from build123d import *

# Parameters (mm, degrees)
F0_W     = 157.5113609433
F0_H     = 71.6332271695
F1_DEPTH = 40
F2_R     = 5
F3_R     = 26.0186453027
F4_DEPTH = 20
F5_W     = 51.7887976021
F5_H     = 11.637929827
F6_DEPTH = 35
F7_R     = 5


# Not quite as in the source:
# - the program builds the solid bodies; features that only make, move or delete a surface that nothing else refers to are left out


with BuildPart() as f1:
    # F0 (on Front) → F1 (new body)
    with BuildSketch(Plane.XZ):
        with Locations((3.7253e-06, 35.8166135848)):
            Rectangle(F0_W, F0_H)
    extrude(amount=F1_DEPTH)

    # F2
    f2_edges = [f1.edges().sort_by_distance(p)[0] for p in [
        (4e-06, -40, 71.633227),
        (4e-06, 0, 71.633227),
        (78.755684, -40, 35.816614),
        (78.755684, 0, 35.816614),
        (78.755684, -20, 71.633227),
        (-78.755677, -20, 71.633227),
        (-78.755677, 0, 35.816614),
        (-78.755677, -40, 35.816614),
    ]]
    fillet(f2_edges, radius=F2_R)

    # F3 (on face) → F4 (cut)
    with BuildSketch(Plane.XZ.offset(40)):
        with Locations((-36.0129252076, 33.036891371)):
            Circle(F3_R)
    extrude(amount=-F4_DEPTH, mode=Mode.SUBTRACT)

    # F5 (on face) → F6 (cut)
    with BuildSketch(Plane.XY.offset(71.6332271695)):
        with Locations((-6.1099091545, -19.590517506)):
            Rectangle(F5_W, F5_H)
    extrude(amount=-F6_DEPTH, mode=Mode.SUBTRACT)

    # F7
    f7_edges = [f1.edges().sort_by_distance(p)[0] for p in [
        (4e-06, -40, 0),
    ]]
    fillet(f7_edges, radius=F7_R)


solid = f1.part
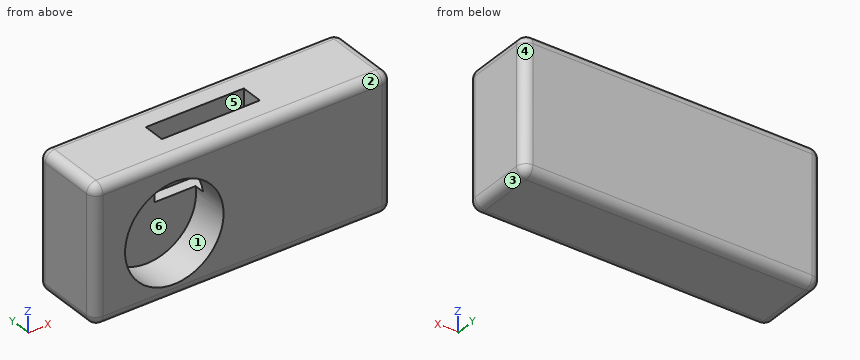
The listing builds one solid part. Answer for the finished solid, in the listing's coordinates (mm). Face numbers are marked on the shaded views. A direction names the side the tool comes from. Give positions to 0.01 mm unless a question says otherwise; leave off trailing zeros. Order: outer loops, then holes, each group sorted by start corner. A loop starts at its lowest first (then second) coordinate and runs counter-clockwise, first axis right, second up. Notation, with made-up numbers: (74.5, 61.25) - (89.5, 61.25) arc R17 cw to (89.5, 88.25) - close; hole circle Ø11 at (-19, 79). An arc over 180 degrees is marked (long way). One line per item, written item: value. Start each with the question number.
1) A cutting plane is placed at C-C on x = -1. Give the vertices of the cut face in (y, z), then the cut area to 3 significant figures.
2) A cutting plane is placed at B-B on y = -33.5. Give the vertices of the cut face in (x, z).
3) The mould has two halves that part along Y. Classify the marked faces 3, 4, 5 and 6: released by +Y, released by -Y, zero draft, split by the parting line, or undercut.
4) Find the intervals of material crossed by L1, parallel to X at y = -19, z = 40; L2, parallel to Y at x = -38.5, z = 13; L3, parallel to X at y = -4.5, z = 38, in increasing order.
5) A tool of negligible diameter and unlimited length cuts with its end or side. For the marked faces 1 and 2, from which of +Z, -Z, +X, -X, +Y, -Y can it reach the whole face along a straight path? Write none if from no direction.
6) Given pin 1 Ø3.5 at (x, y) = (-4.5, -18) entering from +Z; pin 2 Ø5 at (x, z) = (-26.5, 44.5) entering from -Y; pin 3 Ø15.5 at (x, z) = (-25, 31.5) entering from -Y, each flat-ended and moving along its own axis, determine where each tip first touches the part or whether it passes through.
7) A cutting plane is placed at A-A on x = -19.5. Give the vertices of the cut face in (y, z).
8) A cutting plane is placed at D-D on y = -16.5. Give the vertices of the cut face in (x, z).
Answer sheet:
1. outline: (-40, 5) arc R5 ccw to (-35, 0) - (-5, 0) arc R5 ccw to (0, 5) - (0, 66.63) arc R5 ccw to (-5, 71.63) - (-13.77, 71.63) - (-13.77, 36.63) - (-25.41, 36.63) - (-25.41, 71.63) - (-35, 71.63) arc R5 ccw to (-40, 66.63) - close
1. area: 2,440 mm2
2. outline: (-78.76, 5) arc R5 ccw to (-73.76, 0) - (73.76, 0) arc R5 ccw to (78.76, 5) - (78.76, 66.63) arc R5 ccw to (73.76, 71.63) - (-73.76, 71.63) arc R5 ccw to (-78.76, 66.63) - close; hole circle Ø52.04 at (-36.01, 33.04)
3. face 3: zero draft
3. face 4: released by +Y
3. face 5: undercut
3. face 6: released by -Y
4. L1: x = -78.76 to -32, 19.78 to 78.76
4. L2: y = -20 to 0
4. L3: x = -78.73 to 78.73
5. face 1: -Y
5. face 2: +Z, +X, -X, -Y
6. pin 1: stops at z = 36.63
6. pin 2: stops at y = -13.77
6. pin 3: stops at y = -20
7. outline: (-40, 5) arc R5 ccw to (-35, 0) - (-5, 0) arc R5 ccw to (0, 5) - (0, 66.63) arc R5 ccw to (-5, 71.63) - (-13.77, 71.63) - (-13.77, 36.63) - (-20, 36.63) - (-20, 12.93) - (-40, 12.93) - close; (-40, 53.14) - (-25.41, 53.14) - (-25.41, 71.63) - (-35, 71.63) arc R5 ccw to (-40, 66.63) - close
8. outline: (-78.76, 5) arc R5 ccw to (-73.76, 0) - (73.76, 0) arc R5 ccw to (78.76, 5) - (78.76, 66.63) arc R5 ccw to (73.76, 71.63) - (19.78, 71.63) - (19.78, 36.63) - (-32, 36.63) - (-32, 71.63) - (-73.76, 71.63) arc R5 ccw to (-78.76, 66.63) - close
